The listing builds one solid part. Answer for the finished solid, in the listing's coordinates (mm). Face numbers are marked on the shaded views. Round coordinates to 2 decimals unless told otherwise and drop trailing zeros. Loops run counter-clockwise (first coordinate to the right, second up) from the corner with the lowest first, then second, coordinate; pieces in that order, holes last. Notation, with made-up numbers: M 30,43.5 L 56,43.5 A28 ccw 56,70.5 Z; hole C 54,-9.5 d8. An arc over 180 degrees is marked long. Answer as a JSON object with one key per item and string values.
```python
from build123d import *

# Parameters (mm, degrees)
CROQUIS1_R              = 2.5
SALIENTE_EXTRUIR1_DEPTH = 20
REDONDEO1_R             = 2
CROQUIS2_R              = 1.5
CORTAR_EXTRUIR1_DEPTH   = 6
CROQUIS3_R              = 1.5
SALIENTE_EXTRUIR2_DEPTH = 5
REDONDEO2_R             = 2


with BuildPart() as part:
    # Croquis1 → Saliente-Extruir1 (new body)
    with BuildSketch(Plane(origin=(0, 0, 0), x_dir=(1, 0, 0), z_dir=(0, 1, 0))):
        with Locations(Location((0, 0, 0), (0, 0, 270))):
            Circle(CROQUIS1_R)
    extrude(amount=SALIENTE_EXTRUIR1_DEPTH)

    # Redondeo1
    redondeo1_edges = [part.edges().sort_by_distance(p)[0] for p in [
        (0, 0, -2.5),
    ]]
    fillet(redondeo1_edges, radius=REDONDEO1_R)

    # Croquis2 → Cortar-Extruir1 (cut)
    with BuildSketch(Plane.XZ):
        with Locations(Location((0, 0, 0), (0, 0, 270))):
            Circle(CROQUIS2_R)
    extrude(amount=-CORTAR_EXTRUIR1_DEPTH, mode=Mode.SUBTRACT)

    # Croquis3 → Saliente-Extruir2 (add)
    with BuildSketch(Plane(origin=(0, 20, 0), x_dir=(1, 0, 0), z_dir=(0, 1, 0))):
        with Locations(Location((0, 0, 0), (0, 0, 90))):
            Circle(CROQUIS3_R)
    extrude(amount=SALIENTE_EXTRUIR2_DEPTH)

    # Redondeo2
    # the kernel refuses this fillet: 2 mm, written as the material it takes off along each edge
    with BuildSketch(Plane(origin=(0, 20, 0), x_dir=(0, 0, 1), z_dir=(-1, 0, 0))) as redondeo2_piece_1:
        with BuildLine():
            CenterArc((0.5, -1.732050808), REDONDEO2_R, 0, 60)
            Line((1.5, 0), (1.52, 0.034641016))
            ThreePointArc((1.52, 0.034641016), (2, 0.04), (2.5, 0.04))
            Line((2.5, 0.04), (2.54, 0))
            Line((2.54, 0), (2.54, -1.732050808))
            Line((2.54, -1.732050808), (2.5, -1.732050808))
        make_face()
    revolve(axis=Axis((0, 20, 0), (0, 1, 0)), mode=Mode.SUBTRACT)


solid = part.part
```
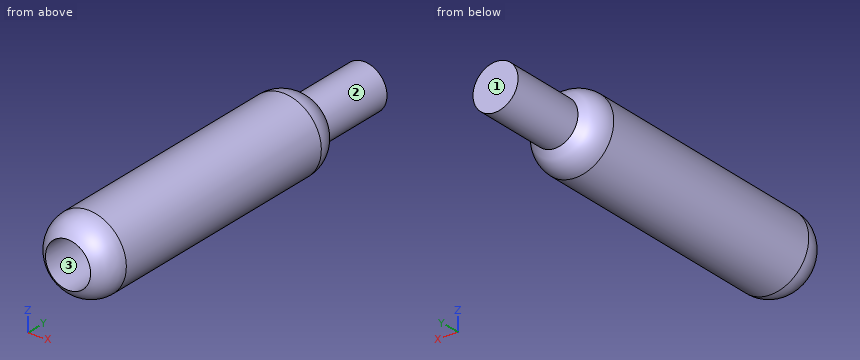
Item 1: The part is cut by section A-A (y = 6.75). Give the vertices of the cut face in (x, z), then the cut area to 3 significant figures.
Values follow:
{"outline": "C 0,0 d5", "area": "19.6 mm^2"}
Item 2: Flat-ended cylindrical pins translate along their axes: P1, Ø1.5, axis at x = -0.5, z = 0, coming from the -Y side; P2, Ø3, axis at y = 9, z = -1.5, coming from the +X side. Find the tip coordinate at first contact, or state that the pin passes through.
Values follow:
{"P1": "y = 6", "P2": "x = 2.5"}
Item 3: Determine the mould class of the marked faces 1, 2 and 3 for opening direction Z: released by +Z, released by -Z, zero draft, split by the parting line, or undercut.
Values follow:
{"face 1": "zero draft", "face 2": "split by the parting line", "face 3": "undercut"}
Item 4: Straight lines are drawn through the part: line 1 (X direction, y = 4.55, z = 0); line 2 (Y direction, x = -1, z = -0.1); line 3 (X direction, y = 22.5, z = -0.1). For each, find the intervals that lie inside material, in ascending order.
Values follow:
{"line 1": "-2.5 to -1.5, 1.5 to 2.5", "line 2": "6 to 25", "line 3": "-1.5 to 1.5"}
